The listing builds one solid part. Answer for the finished solid, in the listing's coordinates (mm). A direction names the side the tool comes from. Coordinates: 2 decimals unless noted, no trailing zeros. Order: outer loops, then holes, each group sorted by start corner. A loop starts at its lowest first (then second) coordinate and runs counter-clockwise, first axis right, second up. Notation, with made-up numbers: (67.25, 10) -> (101.25, 10) arc R6 ccw to (101.25, 21) -> close; hole circle Ø11 at (24, 50). An arc over 180 degrees is marked (long way). Write item = value, one per line. Start each with the question number.
```python
from build123d import *

# Parameters (mm, degrees)
F1_DEPTH = 3.175
F2_W     = 12.7
F2_H     = 3.175
F3_DEPTH = 12.7
F4_R     = 1.6002
F5_R     = 0.7874
F6_DEPTH = 19.377747


with BuildPart() as f1:
    # F0 (on Top) → F1 (new body)
    with BuildSketch(Plane.XY):
        with BuildLine():
            Line((0, 0), (19.05, 0))
            ThreePointArc((19.05, 0), (17.523524, 7.471855), (13.188727, 13.746271))
            ThreePointArc((13.188727, 13.746271), (12.901694, 14.016019), (12.609145, 14.279775))
            ThreePointArc((12.609145, 14.279775), (11.494472, 14.175188), (11.366501, 15.287418))
            ThreePointArc((11.366501, 15.287418), (11.047993, 15.519161), (10.724761, 15.744269))
            ThreePointArc((10.724761, 15.744269), (2.9926, 18.813475), (-5.310256, 18.294908))
            ThreePointArc((-5.310256, 18.294908), (-5.687382, 18.181204), (-6.062075, 18.059727))
            ThreePointArc((-6.062075, 18.059727), (-6.026834, 17.926523), (-6.01497, 17.789247))
            ThreePointArc((-6.01497, 17.789247), (-6.661272, 17.004068), (-7.556042, 17.487388))
            ThreePointArc((-7.556042, 17.487388), (-7.915991, 17.327423), (-8.272556, 17.16005))
            ThreePointArc((-8.272556, 17.16005), (-14.796647, 11.998405), (-18.498984, 4.548637))
            ThreePointArc((-18.498984, 4.548637), (-18.589076, 4.165185), (-18.67122, 3.779952))
            ThreePointArc((-18.67122, 3.779952), (-18.199481, 3.505602), (-18.013375, 2.9926))
            ThreePointArc((-18.013375, 2.9926), (-18.287692, 2.389514), (-18.922543, 2.199969))
            ThreePointArc((-18.922543, 2.199969), (-18.963984, 1.808262), (-18.997317, 1.415781))
            ThreePointArc((-18.997317, 1.415781), (-17.789247, -6.81507), (-13.188727, -13.746271))
            ThreePointArc((-13.188727, -13.746271), (-12.901694, -14.016019), (-12.609145, -14.279775))
            ThreePointArc((-12.609145, -14.279775), (-11.723172, -14.045377), (-11.198305, -14.796647))
            ThreePointArc((-11.198305, -14.796647), (-11.241521, -15.056044), (-11.366501, -15.287418))
            ThreePointArc((-11.366501, -15.287418), (-11.047993, -15.519161), (-10.724761, -15.744269))
            ThreePointArc((-10.724761, -15.744269), (-5.611336, -18.204818), (0, -19.05))
            Line((0, -19.05), (0, 0))
        make_face()
        with BuildLine():
            ThreePointArc((12.609145, 14.279775), (12.901694, 14.016019), (13.188727, 13.746271))
            ThreePointArc((13.188727, 13.746271), (12.998272, 16.029701), (10.724761, 15.744269))
            ThreePointArc((10.724761, 15.744269), (11.047993, 15.519161), (11.366501, 15.287418))
            ThreePointArc((11.366501, 15.287418), (12.257802, 15.553531), (12.798505, 14.796647))
            ThreePointArc((12.798505, 14.796647), (12.749675, 14.521413), (12.609145, 14.279775))
        make_face()
        with BuildLine():
            ThreePointArc((-6.062075, 18.059727), (-5.687382, 18.181204), (-5.310256, 18.294908))
            ThreePointArc((-5.310256, 18.294908), (-7.382992, 19.271685), (-8.272556, 17.16005))
            ThreePointArc((-8.272556, 17.16005), (-7.915991, 17.327423), (-7.556042, 17.487388))
            ThreePointArc((-7.556042, 17.487388), (-7.101303, 18.536396), (-6.062075, 18.059727))
        make_face()
        with BuildLine():
            ThreePointArc((-13.188727, -13.746271), (-12.998272, -16.029701), (-10.724761, -15.744269))
            ThreePointArc((-10.724761, -15.744269), (-11.047993, -15.519161), (-11.366501, -15.287418))
            ThreePointArc((-11.366501, -15.287418), (-12.502338, -15.418106), (-12.609145, -14.279775))
            ThreePointArc((-12.609145, -14.279775), (-12.901694, -14.016019), (-13.188727, -13.746271))
        make_face()
        with BuildLine():
            ThreePointArc((-18.67122, 3.779952), (-18.589076, 4.165185), (-18.498984, 4.548637))
            ThreePointArc((-18.498984, 4.548637), (-20.381265, 3.241984), (-18.997317, 1.415781))
            ThreePointArc((-18.997317, 1.415781), (-18.963984, 1.808262), (-18.922543, 2.199969))
            ThreePointArc((-18.922543, 2.199969), (-19.603641, 3.118289), (-18.67122, 3.779952))
        make_face()
    extrude(amount=F1_DEPTH)

    # F2 (on face) → F3 (join)
    with BuildSketch(Plane.XY.offset(3.175)):
        with Locations((10.828172, 1.5875)):
            Rectangle(F2_W, F2_H)
    extrude(amount=F3_DEPTH)

    # F4
    f4_edges = [f1.edges().sort_by_distance(p)[0] for p in [
        (17.178172, 1.5875, 15.875),
        (4.478172, 1.5875, 15.875),
    ]]
    fillet(f4_edges, radius=F4_R)

    # F5 (on face) → F6 (cut, through all)
    with BuildSketch(Plane.XZ):
        with Locations((15.577972, 14.2748)):
            Circle(F5_R)
        with Locations((6.078372, 14.2748)):
            Circle(F5_R)
    extrude(amount=-F6_DEPTH, mode=Mode.SUBTRACT)


solid = f1.part
```
Item 1: Which of the six approach directions +Z, -Z, +X, -X, +Y, -Y give full straight-line access (tool end or side, diameter ignored) to faces 5 (the flat face through (17.178, 2, 9)), 6 (the flat face through (4.478, 2, 9)), 7 (the flat face through (11, 3.175, 9)), 8 (the flat face through (11, 2, 15.875))?
Item 2: Consider probe 1 along Y at (x, z) = (8.5, 11.5) (3 decimals); probe 2 along X at (y, z) = (-16.5, 0.5). Determine where each line is inside the solid, lowest interval first.
Item 3: Section C-C, the plane y = -9 is taken. Give the vertices of the cut face in (x, z) (3 decimals).
Item 4: Each of these flat-tipped pins is pushed along its axis until it touches: pin 1 (1.5 mm diameter, centred on y = -5, z = 4, fed in from +X); pin 2 (6 mm diameter, centred on y = 1.5, z = 14, fed in from +X); pin 3 (2.5 mm diameter, centred on y = -10, z = 1, fed in from +X); pin 4 (1.8 mm diameter, centred on x = 6.08, z = 14.27, fed in from -Y). Where does it stop, or does it pass through?
Item 5: For a pull along Z with two mould halves and no side action, classify faces 1 (the cylindrical face through (16.722, 1.61, 15.394)), 2 (the flat face through (9, 0, 8)), 3 (the cylindrical face through (16.33, 1.57, 14.51)), 4 (the flat face through (-1, 0, 0)) as pulls with the +Z half, pulls with the -Z half, needs draft (parallel to the pull), parting line crosses it, or undercut.
Item 6: Section A-A, the plane z = 1.75 is taken. Give the number of separate pieces and of enclosed holes in the cut face, then the cut area to 3 significant figures.
Item 7: Section B-B, the plane z = 11.5 is taken. Give the vertices of the cut face in (x, y) (3 decimals), then the cut area to 3 significant figures.
A:
q1.face_5 = +Z, +X, +Y, -Y
q1.face_6 = +Z, -X, +Y, -Y
q1.face_7 = +Z, +X, -X, +Y
q1.face_8 = +Z, +X, -X, +Y, -Y
q2.probe_1 = 0 to 3.175
q2.probe_2 = -9.52 to 0
q3.outline = (-16.79, 0) -> (0, 0) -> (0, 3.175) -> (-16.79, 3.175) -> close
q4.pin_1 = through
q4.pin_2 = 17.18
q4.pin_3 = 0
q4.pin_4 = 0
q5.face_1 = pulls with the +Z half
q5.face_2 = needs draft
q5.face_3 = undercut
q5.face_4 = pulls with the -Z half
q6.separate_pieces = 1
q6.enclosed_holes = 4
q6.area = 863 mm^2
q7.outline = (4.478, 0) -> (17.178, 0) -> (17.178, 3.175) -> (4.478, 3.175) -> close
q7.area = 40.3 mm^2
